Work out the finished part from the listing and answer in its coordinate system (mm). Face numbers are marked on the shaded views. Round coordinates to 2 decimals unless told otherwise and drop trailing zeros. Write each loop counter-clockwise with the first axis right and the second up, starting at its lowest first coordinate (ties: lowest second). Pieces come first, ordered by that corner, then holes. Notation, with made-up numbers: (50, 25.25) - (99, 25.25) arc R21 cw to (99, 64.25) - close; hole circle Ø6 at (27, -37.75). An arc over 180 degrees is marked (long way). Answer as a JSON object with one key per item and string values.
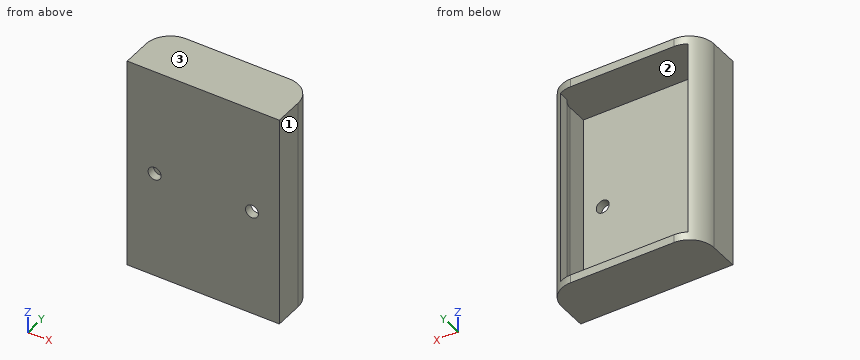
Autodesk Inventor part; units mm, degrees
ref_plane "YZ Plane" through (0, 0, 0) normal (1, 0, 0) x (0, 1, 0)
ref_plane "XZ Plane" through (0, 0, 0) normal (0, 1, 0) x (-1, 0, 0)
ref_plane "XY Plane" through (0, 0, 0) normal (0, 0, 1) x (1, 0, 0)
sketch "スケッチ1" plane through (0, 0, 0) normal (0, 1, 0) x (-1, 0, 0)
  line L0 (-18.75, -26.25) -> (18.75, -26.25)
  line L1 (18.75, -26.25) -> (18.75, 26.25)
  line L2 (18.75, 26.25) -> (-18.75, 26.25)
  line L3 (-18.75, 26.25) -> (-18.75, -26.25)
  line L4 (-18.75, -26.25) -> (18.75, 26.25) construction
  line L5 (18.75, -26.25) -> (-18.75, 26.25) construction
  point P0 (0, 0)
  dimension "d0" = 37.5
  dimension "d1" = 52.5
extrude "押し出し1" add sketch "スケッチ1" along normal blind 13.1
fillet "フィレット1" radius 6 2 edges at (18.75, 13.1, 0) (-18.75, 13.1, 0)
shell "シェル1" thickness 2 removed faces 0
sketch "スケッチ2" plane through (0, 13.1, 0) normal (0, 1, 0) x (1, 0, 0)
  line L0 (16.75, 24.25) -> (-16.75, 24.25)
  line L1 (15.75, -24.25) -> (-15.75, -24.25)
  line L2 (-15.75, -24.25) -> (-15.75, 24.25)
  line L3 (-15.75, 24.25) -> (15.75, 24.25)
  line L4 (15.75, 24.25) -> (15.75, -24.25)
  line L5 (15.75, -24.25) -> (-15.75, 24.25) construction
  line L6 (-15.75, -24.25) -> (15.75, 24.25) construction
  line L7 (-12.75, -26.25) -> (-12.75, 26.25)
  point P0 (0, 0)
  dimension "d8" = 3
extrude "押し出し2" cut sketch "スケッチ2" against normal blind 5
sketch "スケッチ3" plane through (-16.75, 2, 24.25) normal (0, 1, 0) x (1, 0, 0)
  circle A0 centre (28.75, 24.25) radius 1.6
  circle A1 centre (4.75, 24.25) radius 1.6
  line L0 (4, 48.5) -> (29.5, 48.5)
  line L1 (16.75, 48.5) -> (16.75, 0) construction
  line L2 (0, 0) -> (33.5, 0)
  point P0 (16.75, 24.25)
  dimension "d9" = 3.2
  dimension "d11" = 24
extrude "押し出し3" cut sketch "スケッチ3" against normal through all
properties part number "battery_box"
Item 1: A cutting plane is placed at A-A (y = 4.25). Write down the section's boundary in (x, z), and give its area (3 significant figures).
Results found:
{"outline": "(-18.75, -26.25) - (18.75, -26.25) - (18.75, 26.25) - (-18.75, 26.25) - close; hole (-16.75, -24.25) - (16.75, -24.25) - (16.75, 24.25) - (-16.75, 24.25) - close", "area": "344 mm²"}
Item 2: A cutting plane is placed at C-C (z = 0). Write down the section's boundary in (x, y).
Results found:
{"outline": "(-18.75, 0) - (-13.6, 0) - (-13.6, 2) - (-16.75, 2) - (-16.75, 7.1) arc R4 cw to (-15.75, 9.75) - (-15.75, 12.3) arc R6 ccw to (-18.75, 7.1) - close; (-10.4, 0) - (10.4, 0) - (10.4, 2) - (-10.4, 2) - close; (13.6, 0) - (18.75, 0) - (18.75, 7.1) arc R6 ccw to (15.75, 12.3) - (15.75, 9.75) arc R4 cw to (16.75, 7.1) - (16.75, 2) - (13.6, 2) - close"}
Item 3: Each of these flat-tipped pins is pushed along its axis until it touches: P1, Ø10, axis at x = -9, z = -14.5, coming from the +Y side; P2, Ø2, axis at y = 11.5, z = 5, coming from the +X side; P3, Ø3, axis at y = 10, z = -8.5, coming from the -X side. Where does it stop, or does it pass through?
Results found:
{"P1": "y = 2", "P2": "x = 17.69", "P3": "x = -18.58"}
Item 4: Consider line 1 along X through (y, z) = (0.7, 0); line 2 along X through (y, z) = (2.75, -20.5); line 3 along Z through (x, y) = (-13, 5). Determine where each line is inside the solid, lowest interval first.
Results found:
{"line 1": "-18.75 to -13.6, -10.4 to 10.4, 13.6 to 18.75", "line 2": "-18.75 to -16.75, 16.75 to 18.75", "line 3": "-26.25 to -24.25, 24.25 to 26.25"}
Item 5: A cutting plane is placed at B-B (x = 12). Write down the section's boundary in (y, z).
Results found:
{"outline": "(0, -26.25) - (13.1, -26.25) - (13.1, -24.25) - (2, -24.25) - (2, -1.6) - (0, -1.6) - close; (0, 1.6) - (2, 1.6) - (2, 24.25) - (13.1, 24.25) - (13.1, 26.25) - (0, 26.25) - close"}
Item 6: A cutting plane is placed at D-D (z = 13.5). Write down the section's boundary in (x, y), and give its area (3 significant figures).
Results found:
{"outline": "(-18.75, 0) - (18.75, 0) - (18.75, 7.1) arc R6 ccw to (15.75, 12.3) - (15.75, 9.75) arc R4 cw to (16.75, 7.1) - (16.75, 2) - (-16.75, 2) - (-16.75, 7.1) arc R4 cw to (-15.75, 9.75) - (-15.75, 12.3) arc R6 ccw to (-18.75, 7.1) - close", "area": "114 mm²"}
Item 7: Determine the mould class of the marked faces 1, 2 and 3 for opening direction X: pulls with the +X half, pulls with the -X half, needs draft (parallel to the pull), parting line crosses it, or undercut.
Results found:
{"face 1": "pulls with the +X half", "face 2": "undercut", "face 3": "needs draft"}
